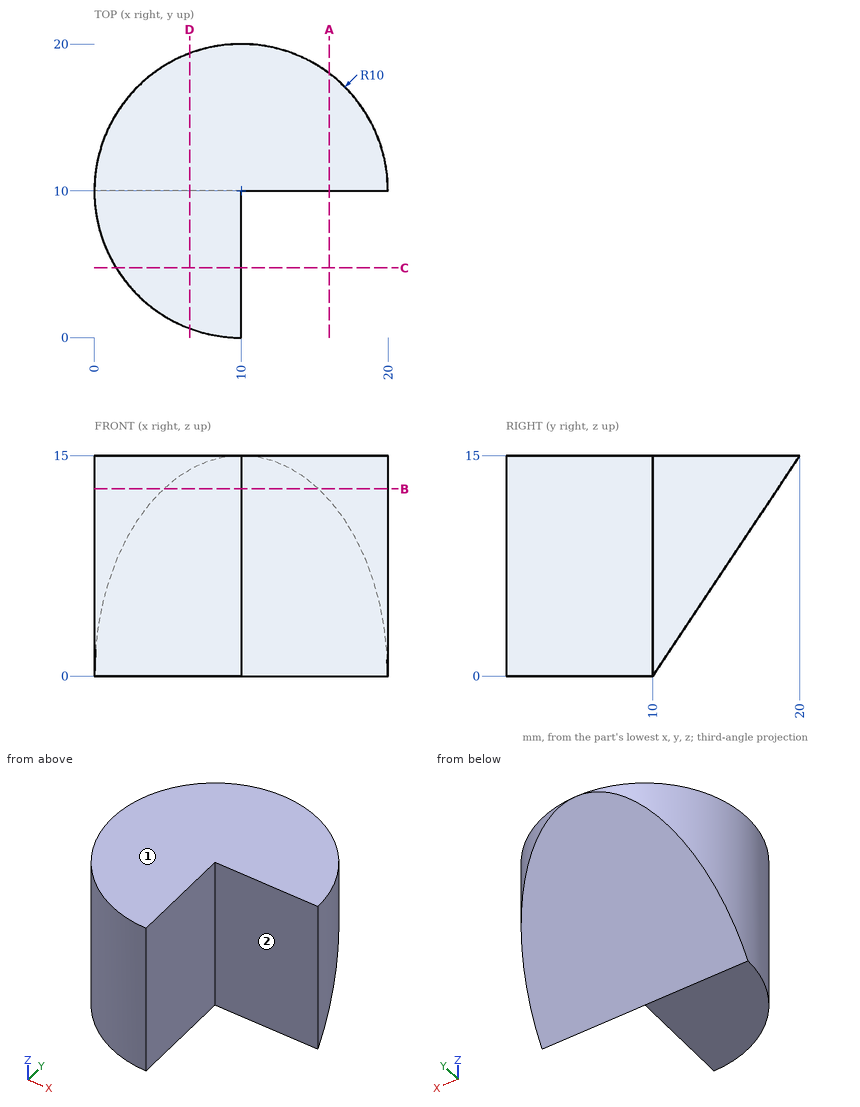
Here's the drawing with two shaded views (mm, measured from the low corner). I have some questions. A direction names the side the tool comes from. Round coordinates to 2 decimals unless told otherwise and drop trailing zeros. Order: outer loops, then holes, each group sorted by start corner. A loop starts at its lowest first (then second) coordinate and runs counter-clockwise, first axis right, second up. Notation, with made-up numbers: (37, -17) -> (74, -17) arc R24 cw to (74, 0) -> close; hole circle Ø4 at (26.5, 14). An arc over 180 degrees is marked (long way). Use a Markdown table: item, result. Add a question column.
(1) I need wall thicknesses on line 1 along Y through (x, z) = (2.5, 11); line 2 along Z through (x, y) = (9, 17); line 3 along Y through (x, z) = (12, 7.75). Which ranges of each line are inside material? Lowest first, please.
(2) For pin 1 Ø5 at (x, z) = (16, 12) entering from +Y; pin 2 Ø8 at (x, z) = (16, 4.5) entering from -Y; pin 3 Ø1.5 at (x, y) = (14, 9) entering from +Z; pin 4 Ø4 at (y, z) = (6, 5) entering from +X, each with a flat end and sliding along its axis, tell me the tip position at first contact or that it passes through.
(3) For the marked faces 1 and 2, which set-ups out of +Z, -Z, +X, -X, +Y, -Y let a thin tool reach every point of the face, with its end or its side?
(4) Suppose I cut it at C-C, the plane y = 4.75. Please give me the cut outline in (x, z), and give its area (3 significant figures).
(5) Suppose I cut it at B-B, the plane z = 12.75. Please give me the cut outline in (x, y).
(6) Suppose I cut it at A-A, the plane x = 16. Please give me the cut outline in (y, z).
(7) Suppose I cut it at D-D, the plane x = 6.5. Please give me the cut outline in (y, z), and give its area (3 significant figures).
Verdict:
| question | item | result |
|---|---|---|
| 1 | line 1 | 3.39 to 16.61 |
| 1 | line 2 | 10.5 to 15 |
| 1 | line 3 | 10 to 15.17 |
| 2 | pin 1 | y = 19.11 |
| 2 | pin 2 | y = 10 |
| 2 | pin 3 | through |
| 2 | pin 4 | x = 10 |
| 3 | face 1 | +Z, +X, -X, +Y, -Y |
| 3 | face 2 | +Z, -Z, +X, -Y |
| 4 | outline | (1.49, 0) -> (10, 0) -> (10, 15) -> (1.49, 15) -> close |
| 4 | area | 128 mm2 |
| 5 | outline | (4.73, 18.5) arc R10 ccw to (10, 0) -> (10, 10) -> (20, 10) arc R10 ccw to (15.27, 18.5) -> close |
| 6 | outline | (10, 0) -> (18, 12) -> (18, 15) -> (10, 15) -> close |
| 7 | outline | (0.63, 0) -> (10, 0) -> (19.37, 14.05) -> (19.37, 15) -> (0.63, 15) -> close |
| 7 | area | 215 mm2 |
